from build123d import *

# Parameters (mm, degrees)
F0_W     = 20.32
F0_H     = 152.4
F1_DEPTH = 1.27
F2_W     = 20.32
F2_H     = 2.54
F3_DEPTH = 3.81
F4_W     = 1.27
F4_H     = 50.8
F5_DEPTH = 5.08


with BuildPart() as f1:
    # F0 (on Front) → F1 (new body)
    with BuildSketch(Plane.XZ):
        with Locations((10.16, 76.2)):
            Rectangle(F0_W, F0_H)
    extrude(amount=F1_DEPTH)

    # F2 (on face) → F3 (join)
    with BuildSketch(Plane.XZ.offset(1.27)):
        with Locations((10.16, 1.27)):
            Rectangle(F2_W, F2_H)
    extrude(amount=F3_DEPTH)

    # F4 (on face) → F5 (join)
    with BuildSketch(Plane(origin=(0, 0, 0), x_dir=(-1, 0, 0), z_dir=(0, 1, 0))):
        with Locations((-0.635, 127)):
            Rectangle(F4_W, F4_H)
        with Locations((-19.685, 127)):
            Rectangle(F4_W, F4_H)
    extrude(amount=F5_DEPTH)


solid = f1.part
Read the model definition and answer for the solid it produces. Units are mm, in the model's axes. A direction names the side the tool comes from. Coordinates: 2 decimals unless noted, no trailing zeros. Order: outer loops, then holes, each group sorted by start corner. A loop starts at its lowest first (then second) coordinate and runs counter-clockwise, first axis right, second up. Notation, with made-up numbers: M 37.25,-32 L 62.25,-32 A5 cw 62.25,-24 Z; hole C -3.75,53 d9. An arc over 180 degrees is marked long. Put each result on its own line as item: value. Start each with the question number.
Item 1: Section B-B, the plane x = 5 is taken. Determine the outline of the cut face in (y, z), plus the area to 3 significant figures.
Item 2: Section C-C, the plane z = 126.5 is taken. Determine the outline of the cut face in (x, y), plus the area to 3 significant figures.
Item 3: Given pin 1 Ø5 at (x, z) = (11.5, 93) entering from +Y; pin 2 Ø3 at (x, y) = (5.5, -3.5) entering from +Z; pin 3 Ø0.6 at (x, y) = (0.5, 2) entering from -Z, each flat-ended and moving along its own axis, determine where each tip first touches the part or whether it passes through.
Item 4: Section D-D, the plane y = -3.75 is taken. Determine the outline of the cut face in (x, z), plus the area to 3 significant figures.
Item 5: For faces 1 (the face through (1.27, 3, 127)), 2 (the face through (10, -3, 0)), 3 (the face through (10, -1.27, 79)), determine the directions among +Z, -Z, +X, -X, +Y, -Y from which every point of the face is accessible in a straight line to the end or side of a thin tool.
Item 6: Consider probe 1 along Y at (x, z) = (1.75, 123.5); probe 2 along Z at (x, y) = (6.25, -4); probe 3 along Z at (x, y) = (19.5, 3.75). Determine where each line is inside the solid, lowest interval first. Write a range as [from, to].
Item 7: Section A-A, the plane y = 3.75 is taken. Determine the outline of the cut face in (x, z), plus the area to 3 significant figures.
Item 8: The mould has two halves that part along X. Classify faces 4 (the face through (19.05, 3, 127)), 5 (the face through (20.32, 1, 104)), 6 (the face through (10, -5.08, 1)): +X half, -X half, draft (parallel to the pull), parting line (faces both ways), or undercut.
Computed:
1. outline: M -5.08,0 L 0,0 L 0,152.4 L -1.27,152.4 L -1.27,2.54 L -5.08,2.54 Z
1. area: 203 mm2
2. outline: M 0,-1.27 L 20.32,-1.27 L 20.32,5.08 L 19.05,5.08 L 19.05,0 L 1.27,0 L 1.27,5.08 L 0,5.08 Z
2. area: 38.7 mm2
3. pin 1: stops at y = 0
3. pin 2: stops at z = 2.54
3. pin 3: stops at z = 101.6
4. outline: M 0,0 L 20.32,0 L 20.32,2.54 L 0,2.54 Z
4. area: 51.6 mm2
5. face 1: +Z, -Z, +Y
5. face 2: -Z, +X, -X, +Y, -Y
5. face 3: +Z, +X, -X, -Y
6. probe 1: y = [-1.27, 0]
6. probe 2: z = [0, 2.54]
6. probe 3: z = [101.6, 152.4]
7. outline: M 0,101.6 L 1.27,101.6 L 1.27,152.4 L 0,152.4 Z; M 19.05,101.6 L 20.32,101.6 L 20.32,152.4 L 19.05,152.4 Z
7. area: 129 mm2
8. face 4: undercut
8. face 5: +X half
8. face 6: draft
